```python
from build123d import *

# Parameters (mm, degrees)
BOSS_EXTRUDE1_DEPTH     = 125
SKETCH2_R               = 3
CUT_EXTRUDE1_DEPTH      = 6
CUT_EXTRUDE1_DEPTH_BACK = 6


with BuildPart() as part:
    # Sketch1 → Boss-Extrude1 (new body, symmetric)
    with BuildSketch(Plane(origin=(0, 0, 0), x_dir=(0, 0, -1), z_dir=(1, 0, 0))):
        Polygon((0, 5.773502692), (-5, 2.886751346), (-5, -2.886751346), (0, -5.773502692), (5, -2.886751346), (5, 2.886751346), align=None)
    extrude(amount=BOSS_EXTRUDE1_DEPTH, both=True)

    # Sketch2 → Cut-Extrude1 (cut, two sides)
    with BuildSketch(Plane.XY) as cut_extrude1_sk:
        with Locations((115, 0)):
            Circle(SKETCH2_R)
        with Locations((-115, 0)):
            Circle(SKETCH2_R)
        with Locations((-65, 0)):
            Circle(SKETCH2_R)
    extrude(amount=CUT_EXTRUDE1_DEPTH, mode=Mode.SUBTRACT)
    extrude(cut_extrude1_sk.sketch, amount=-CUT_EXTRUDE1_DEPTH_BACK, mode=Mode.SUBTRACT)


solid = part.part
```
CAD build for the part. Positions are in the model's coordinates, mm. Round coordinates to 2 decimals unless told otherwise and drop trailing zeros. Order: outer loops, then holes, each group sorted by start corner. A loop starts at its lowest first (then second) coordinate and runs counter-clockwise, first axis right, second up. Notation, with made-up numbers: (9, 28.5) - (37, 28.5) arc R18 ccw to (37, 62.5) - close; hole circle Ø3 at (-25, -34). An arc over 180 degrees is marked (long way). Use CSV: the item, a comma, the result in double quotes. Start each with the question number.
1) Saw through at C-C (x = 3.5). List the corners of the cut face in (y, z), and give its area (3 significant figures).
2) Wall check: L1, parallel to X at y = 0, z = -3.2; L2, parallel to Y at x = 115, z = 1.05; L3, parallel to Y at x = 115, z = 2.5. Give the ranges that are in metal, low to high. Write a range as [from, to].
3) Saw through at A-A (y = 0). List the corners of the cut face in (x, z), and give its area (3 significant figures).
4) Pin check, flat tips, straight feed: pin 1 Ø4 at (y, z) = (-4, -3.5) entering from +X; pin 2 Ø1.5 at (x, z) = (-97, -3.5) entering from -Y. Stop position of each tip, or through.
5) Saw through at B-B (z = 2.5). List the corners of the cut face in (x, y), and give its area (3 significant figures).
Values follow:
1,outline,"(-5.77, 0) - (-2.89, -5) - (2.89, -5) - (5.77, 0) - (2.89, 5) - (-2.89, 5) - close"
1,area,"86.6 mm2"
2,L1,"x = [-125, -118], [-112, -68], [-62, 112], [118, 125]"
2,L2,"y = [-5.17, -3], [3, 5.17]"
2,L3,"y = [-4.33, -3], [3, 4.33]"
3,outline,"(-125, -5) - (-118, -5) - (-118, 5) - (-125, 5) - close; (-112, -5) - (-68, -5) - (-68, 5) - (-112, 5) - close; (-62, -5) - (112, -5) - (112, 5) - (-62, 5) - close; (118, -5) - (125, -5) - (125, 5) - (118, 5) - close"
3,area,"2,320 mm2"
4,pin 1,"stops at x = 125"
4,pin 2,"stops at y = -4.19"
5,outline,"(-125, -4.33) - (125, -4.33) - (125, 4.33) - (-125, 4.33) - close; hole circle Ø6 at (-115, 0); hole circle Ø6 at (-65, 0); hole circle Ø6 at (115, 0)"
5,area,"2,080 mm2"
